Verification items for the finished model (mm, model axes). A direction names the side the tool comes from. Coordinates: 2 decimals unless noted, no trailing zeros. Write each loop counter-clockwise with the first axis right and the second up, starting at its lowest first coordinate (ties: lowest second). Pieces come first, ordered by that corner, then holes. Notation, with made-up numbers: (20, 44.25) -> (63, 44.25) arc R28 cw to (63, 78.25) -> close; hole circle Ø2 at (-3.5, -27). An arc over 180 degrees is marked (long way). Answer in a Markdown table with one row per item.
```python
from build123d import *

# Parameters (mm, degrees)
SKETCH1_R           = 30
SKETCH1_R_2         = 15
BOSS_EXTRUDE1_DEPTH = 10
CUT_EXTRUDE1_DEPTH  = 43
SKETCH4_R           = 1
CUT_EXTRUDE3_DEPTH  = 43
SKETCH5_R           = 1
CUT_EXTRUDE4_DEPTH  = 70
SKETCH6_R           = 1
CUT_EXTRUDE5_DEPTH  = 70
SKETCH8_R           = 2.5
CUT_EXTRUDE6_DEPTH  = 4
SKETCH9_R           = 2.5
SKETCH9_R_2         = 1
CUT_EXTRUDE7_DEPTH  = 4
SKETCH10_R          = 2.5
CUT_EXTRUDE8_DEPTH  = 4
SKETCH11_R          = 2.5
CUT_EXTRUDE9_DEPTH  = 4


with BuildPart() as part:
    # Sketch1 → Boss-Extrude1 (new body)
    with BuildSketch(Plane(origin=(0, 0, 0), x_dir=(1, 0, 0), z_dir=(0, 1, 0))):
        Circle(SKETCH1_R)
        Circle(SKETCH1_R_2, mode=Mode.SUBTRACT)
    extrude(amount=BOSS_EXTRUDE1_DEPTH)

    # Sketch2 → Cut-Extrude1 (cut)
    with BuildSketch(Plane(origin=(0, 10, 0), x_dir=(1, 0, 0), z_dir=(0, 1, 0))):
        with BuildLine():
            ThreePointArc((10.770329614, 28), (0, 30), (-10.770329614, 28))
            Line((-10.770329614, 28), (10.770329614, 28))
        make_face()
        with BuildLine():
            Line((-28, -10.770329614), (-28, 10.770329614))
            ThreePointArc((-28, 10.770329614), (-30, 0), (-28, -10.770329614))
        make_face()
        with BuildLine():
            ThreePointArc((30, 0), (29.495762408, 5.477225575), (28, 10.770329614))
            Line((28, 10.770329614), (28, -10.770329614))
            ThreePointArc((28, -10.770329614), (29.495762408, -5.477225575), (30, 0))
        make_face()
        with BuildLine():
            Line((10.770329614, -28), (-10.770329614, -28))
            ThreePointArc((-10.770329614, -28), (0, -30), (10.770329614, -28))
        make_face()
    extrude(amount=-CUT_EXTRUDE1_DEPTH, mode=Mode.SUBTRACT)

    # Sketch4 → Cut-Extrude3 (cut)
    with BuildSketch(Plane(origin=(0, 10, 0), x_dir=(1, 0, 0), z_dir=(0, 1, 0))):
        with Locations((15.909902577, -15.909902577)):
            Circle(SKETCH4_R)
        with Locations((-15.909902577, -15.909902577)):
            Circle(SKETCH4_R)
        with Locations((-15.909902577, 15.909902577)):
            Circle(SKETCH4_R)
        with Locations((15.909902577, 15.909902577)):
            Circle(SKETCH4_R)
    extrude(amount=-CUT_EXTRUDE3_DEPTH, mode=Mode.SUBTRACT)

    # Sketch5 → Cut-Extrude4 (cut)
    with BuildSketch(Plane(origin=(0, 0, -28), x_dir=(-1, 0, 0), z_dir=(0, 0, -1))):
        with Locations((0, 5)):
            Circle(SKETCH5_R)
    extrude(amount=-CUT_EXTRUDE4_DEPTH, mode=Mode.SUBTRACT)

    # Sketch6 → Cut-Extrude5 (cut)
    with BuildSketch(Plane(origin=(28, 0, 0), x_dir=(0, 0, -1), z_dir=(1, 0, 0))):
        with Locations((-0.045783142, 5)):
            Circle(SKETCH6_R)
    extrude(amount=-CUT_EXTRUDE5_DEPTH, mode=Mode.SUBTRACT)

    # Sketch8 → Cut-Extrude6 (cut)
    with BuildSketch(Plane(origin=(0, 0, -28), x_dir=(-1, 0, 0), z_dir=(0, 0, -1))):
        with Locations((0, 5)):
            Circle(SKETCH8_R)
    extrude(amount=-CUT_EXTRUDE6_DEPTH, mode=Mode.SUBTRACT)

    # Sketch9 → Cut-Extrude7 (cut)
    with BuildSketch(Plane(origin=(28, 0, 0), x_dir=(0, 0, -1), z_dir=(1, 0, 0))):
        with Locations((-0.045783142, 5)):
            Circle(SKETCH9_R)
        with Locations((-0.045783142, 5)):
            Circle(SKETCH9_R_2, mode=Mode.SUBTRACT)
    extrude(amount=-CUT_EXTRUDE7_DEPTH, mode=Mode.SUBTRACT)

    # Sketch10 → Cut-Extrude8 (cut)
    with BuildSketch(Plane.XY.offset(28)):
        with Locations((0, 5)):
            Circle(SKETCH10_R)
    extrude(amount=-CUT_EXTRUDE8_DEPTH, mode=Mode.SUBTRACT)

    # Sketch11 → Cut-Extrude9 (cut)
    with BuildSketch(Plane.ZY.offset(28)):
        with Locations((0.045783142, 5)):
            Circle(SKETCH11_R)
    extrude(amount=-CUT_EXTRUDE9_DEPTH, mode=Mode.SUBTRACT)


solid = part.part
```
1. Go/stop test with flat-tipped pins: pin 1 (1.8 mm diameter, centred on x = -15.91, z = 15.91, fed in from +Y); pin 2 (5 mm diameter, centred on x = 22, y = 7, fed in from +Z); pin 3 (4 mm diameter, centred on y = 6, z = 16.5, fed in from +X); pin 4 (5.5 mm diameter, centred on x = -0.5, y = 4, fed in from +Z). Record where each tip stops, or that it passes through.
Findings below:
| item | result |
|---|---|
| pin 1 | passes through |
| pin 2 | stops at z = 22.8 |
| pin 3 | stops at x = 26.26 |
| pin 4 | stops at z = 28 |
2. Sectioned sample at B-B, the plane y = 9. Record the cut outline in (x, z).
Findings below:
| item | result |
|---|---|
| outline | (-28, -10.77) arc R30 ccw to (-10.77, -28) -> (10.77, -28) arc R30 ccw to (28, -10.77) -> (28, 10.77) arc R30 ccw to (10.77, 28) -> (-10.77, 28) arc R30 ccw to (-28, 10.77) -> close; hole circle Ø2 at (-15.91, -15.91); hole circle Ø2 at (-15.91, 15.91); hole circle Ø30 at (0, 0); hole circle Ø2 at (15.91, -15.91); hole circle Ø2 at (15.91, 15.91) |
3. Sectioned sample at A-A, the plane x = 0. Record the cut outline in (y, z), and give its area (3 significant figures).
Findings below:
| item | result |
|---|---|
| outline | (0, -28) -> (2.5, -28) -> (2.5, -24) -> (4, -24) -> (4, -15) -> (0, -15) -> close; (0, 15) -> (4, 15) -> (4, 24) -> (2.5, 24) -> (2.5, 28) -> (0, 28) -> close; (6, -24) -> (7.5, -24) -> (7.5, -28) -> (10, -28) -> (10, -15) -> (6, -15) -> close; (6, 15) -> (10, 15) -> (10, 28) -> (7.5, 28) -> (7.5, 24) -> (6, 24) -> close |
| area | 184 mm² |
4. Sectioned sample at D-D, the plane x = -6.5. Record the cut outline in (y, z), and give its area (3 significant figures).
Findings below:
| item | result |
|---|---|
| outline | (0, -28) -> (10, -28) -> (10, -13.52) -> (0, -13.52) -> close; (0, 13.52) -> (10, 13.52) -> (10, 28) -> (0, 28) -> close |
| area | 290 mm² |
5. Release check for a two-part mould opening along Z. For faces 5 (the face through (-24, 4, 1)), 6 (the face through (21.337, 4.93, -21.089)), 7 (the face through (0, 6, 19)) record: released by +Z, released by -Z, zero draft, split by the parting line, or undercut.
Findings below:
| item | result |
|---|---|
| face 5 | undercut |
| face 6 | released by -Z |
| face 7 | zero draft |
6. Sectioned sample at C-C, the plane z = 0. Record the cut outline in (x, y), and give its area (3 significant figures).
Findings below:
| item | result |
|---|---|
| outline | (-28, 0) -> (-15, 0) -> (-15, 4) -> (-24, 4) -> (-24, 2.5) -> (-28, 2.5) -> close; (-28, 7.5) -> (-24, 7.5) -> (-24, 6) -> (-15, 6) -> (-15, 10) -> (-28, 10) -> close; (15, 0) -> (28, 0) -> (28, 2.5) -> (24, 2.5) -> (24, 4) -> (15, 4) -> close; (15, 6) -> (24, 6) -> (24, 7.5) -> (28, 7.5) -> (28, 10) -> (15, 10) -> close |
| area | 184 mm² |
7. Access from +Z, -Z, +X, -X, +Y, -Y to the whole of each face (thin tool, end or side, straight path). Record for faces 1 (the face through (24, 4, -1)), 2 (the face through (-26.03, 7.48, -0.28)), 3 (the face through (0.33, 7.48, -26.03)), 4 (the face through (-13, 0, -13)).
Findings below:
| item | result |
|---|---|
| face 1 | +X |
| face 2 | -X |
| face 3 | -Z |
| face 4 | +Z, -Z, +X, -X, -Y |
8. Material ranges on probe 1 along Z at (x, y) = (1.5, 9.5); probe 2 along Z at (x, y) = (-15.5, 3.5); probe 3 along X at (y, z) = (2, -16.5), recorded low to high. Write a range as from..to.
Findings below:
| item | result |
|---|---|
| probe 1 | z = -28..-14.92, 14.92..28 |
| probe 2 | z = -25.69..-16.82, -15..15, 16.82..25.69 |
| probe 3 | x = -25.05..-16.72, -15.1..15.1, 16.72..25.05 |
